Work out the finished part from the listing and answer in its coordinate system (mm). Round coordinates to 2 decimals unless told otherwise and drop trailing zeros. Loops run counter-clockwise (first coordinate to the right, second up) from the corner with the lowest first, then second, coordinate; pieces in that order, holes last. Notation, with made-up numbers: (1, 1.25) - (56, 1.25) arc R17 cw to (56, 23.25) - close; hole circle Ø5 at (21.25, 73). An arc over 180 degrees is marked (long way). Answer as CSV lines item,"result". Start each with the question number.
Q1. Section A-A on x = 0 is taken. Write down the section's boundary in (y, z), then the cut area to 3 significant figures.
Q2. Section B-B on z = 0.7 is taken. Write down the section's boundary in (x, y), then the cut area to 3 significant figures.
Q3. This flat-tipped pin is pushed along its axis until it touches: pin 1 Ø0.8 at (x, z) = (41.5, 0.5) entering from +Y. Where does it stop, or does it pass through?
Q4. Straight lines are drawn through the part: L1, parallel to Y at x = 0, z = 0.6; L2, parallel to X at y = -23, z = 0.4; L3, parallel to Y at x = 13, z = 0.45. For each, find the intervals that lie inside material, in ascending order. Write a range as [from, to].
Q5. Section C-C on y = -12.5 is taken. Write down the section's boundary in (x, z).
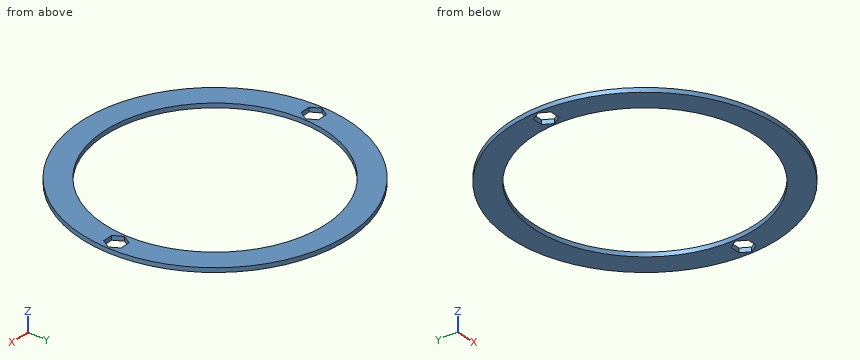
```python
from build123d import *

# Parameters (mm, degrees)
ESQUISSE1_R        = 46.25
ESQUISSE1_R_2      = 38.25
BOSS_EXTRU_1_DEPTH = 1.5


with BuildPart() as part:
    # Esquisse1 → Boss.-Extru.1 (new body)
    with BuildSketch(Plane.XY):
        Circle(ESQUISSE1_R)
        Circle(ESQUISSE1_R_2, mode=Mode.SUBTRACT)
        Polygon((-40.517949192, 3), (-43.982050808, 3), (-45.714101615, 0), (-43.982050808, -3), (-40.517949192, -3), (-38.785898385, 0), align=None, mode=Mode.SUBTRACT)
        Polygon((38.785898385, 0), (40.517949192, 3), (43.982050808, 3), (45.714101615, 0), (43.982050808, -3), (40.517949192, -3), align=None, mode=Mode.SUBTRACT)
    extrude(amount=BOSS_EXTRU_1_DEPTH)


solid = part.part
```
Findings:
1,outline,"(-46.25, 0) - (-38.25, 0) - (-38.25, 1.5) - (-46.25, 1.5) - close; (38.25, 0) - (46.25, 0) - (46.25, 1.5) - (38.25, 1.5) - close"
1,area,"24.0 mm^2"
2,outline,"circle Ø92.5 at (0, 0); hole (-45.71, 0) - (-43.98, -3) - (-40.52, -3) - (-38.79, 0) - (-40.52, 3) - (-43.98, 3) - close; hole circle Ø76.5 at (0, 0); hole (38.79, 0) - (40.52, -3) - (43.98, -3) - (45.71, 0) - (43.98, 3) - (40.52, 3) - close"
2,area,"2,060 mm^2"
3,pin 1,"stops at y = 21.21"
4,L1,"y = [-46.25, -38.25], [38.25, 46.25]"
4,L2,"x = [-40.13, -30.56], [30.56, 40.13]"
4,L3,"y = [-44.39, -35.97], [35.97, 44.39]"
5,outline,"(-44.53, 0) - (-36.15, 0) - (-36.15, 1.5) - (-44.53, 1.5) - close; (36.15, 0) - (44.53, 0) - (44.53, 1.5) - (36.15, 1.5) - close"
